For this review, take the finished solid that the model builds, in its own axes (mm). A direction names the side the tool comes from. Give positions to 0.01 mm unless a question says otherwise; leave off trailing zeros. Order: outer loops, then holes, each group sorted by start corner. A loop starts at its lowest first (then second) coordinate and runs counter-clockwise, first axis right, second up.
from build123d import *

# Parameters (mm, degrees)
F0_W     = 70
F0_H     = 50
F0_W_2   = 2.8157552083
F0_H_2   = 18.5818142361
F0_R     = 2.5
F1_DEPTH = 5


with BuildPart() as f1:
    # F0 (on Top) → F1 (new body)
    with BuildSketch(Plane.XY):
        with Locations((-35, 25)):
            Rectangle(F0_W, F0_H)
        Polygon((-58.9236111111, 34.7884114583), (-52.3589409722, 22.3914930556), (-45.7508680556, 34.7884114583), (-42.6312934028, 34.7884114583), (-50.9049479167, 19.6137152778), (-50.9049479167, 10), (-53.818359375, 10), (-53.818359375, 19.4780815972), (-62.0757378472, 34.7884114583), align=None, mode=Mode.SUBTRACT)
        with BuildLine():
            Line((-26.1328125, 10), (-28.2215711806, 10))
            Line((-28.2215711806, 10), (-28.7803819444, 12.6475694444))
            Line((-28.7803819444, 12.6475694444), (-28.916015625, 12.6475694444))
            add(Edge.make_bspline(
                [(-28.916015625, 12.6475694444), (-30.3049045139, 10.9006076389), (-31.6856553819, 10.2794053819)],
                knots=[0, 0, 0, 1, 1, 1], degree=2))
            add(Edge.make_bspline(
                [(-31.6856553819, 10.2794053819), (-33.06640625, 9.658203125), (-35.1388888889, 9.658203125)],
                knots=[0, 0, 0, 1, 1, 1], degree=2))
            add(Edge.make_bspline(
                [(-35.1388888889, 9.658203125), (-37.900390625, 9.658203125), (-39.4683159722, 11.0850694444)],
                knots=[0, 0, 0, 1, 1, 1], degree=2))
            add(Edge.make_bspline(
                [(-39.4683159722, 11.0850694444), (-41.0362413194, 12.5119357639), (-41.0362413194, 15.1378038194)],
                knots=[0, 0, 0, 1, 1, 1], degree=2))
            add(Edge.make_bspline(
                [(-41.0362413194, 15.1378038194), (-41.0362413194, 20.7638888889), (-32.0355902778, 21.03515625)],
                knots=[0, 0, 0, 1, 1, 1], degree=2))
            Line((-32.0355902778, 21.03515625), (-28.8834635417, 21.1382378472))
            Line((-28.8834635417, 21.1382378472), (-28.8834635417, 22.2938368056))
            add(Edge.make_bspline(
                [(-28.8834635417, 22.2938368056), (-28.8834635417, 24.4802517361), (-29.8220486111, 25.5219184028)],
                knots=[0, 0, 0, 1, 1, 1], degree=2))
            add(Edge.make_bspline(
                [(-29.8220486111, 25.5219184028), (-30.7606336806, 26.5635850694), (-32.8331163194, 26.5635850694)],
                knots=[0, 0, 0, 1, 1, 1], degree=2))
            add(Edge.make_bspline(
                [(-32.8331163194, 26.5635850694), (-35.1551649306, 26.5635850694), (-38.0848524306, 25.1421440972)],
                knots=[0, 0, 0, 1, 1, 1], degree=2))
            Line((-38.0848524306, 25.1421440972), (-38.9529079861, 27.2960069444))
            add(Edge.make_bspline(
                [(-38.9529079861, 27.2960069444), (-37.5802951389, 28.0392795139), (-35.9445529514, 28.4624565972)],
                knots=[0, 0, 0, 1, 1, 1], degree=2))
            add(Edge.make_bspline(
                [(-35.9445529514, 28.4624565972), (-34.3088107639, 28.8856336806), (-32.6595052083, 28.8856336806)],
                knots=[0, 0, 0, 1, 1, 1], degree=2))
            add(Edge.make_bspline(
                [(-32.6595052083, 28.8856336806), (-29.3391927083, 28.8856336806), (-27.7360026042, 27.4126519097)],
                knots=[0, 0, 0, 1, 1, 1], degree=2))
            add(Edge.make_bspline(
                [(-27.7360026042, 27.4126519097), (-26.1328125, 25.9396701389), (-26.1328125, 22.6844618056)],
                knots=[0, 0, 0, 1, 1, 1], degree=2))
            Line((-26.1328125, 22.6844618056), (-26.1328125, 10))
        make_face(mode=Mode.SUBTRACT)
        with Locations((-18.9306640625, 19.2909071181)):
            Rectangle(F0_W_2, F0_H_2, mode=Mode.SUBTRACT)
        with Locations((-41.0378689236, 42.0710678119)):
            Circle(F0_R, mode=Mode.SUBTRACT)
        with BuildLine():
            add(Edge.make_bspline(
                [(-20.1025390625, 32.2005208333), (-20.5772569444, 32.6671006944), (-20.5772569444, 33.6165364583)],
                knots=[0, 0, 0, 1, 1, 1], degree=2))
            add(Edge.make_bspline(
                [(-20.5772569444, 33.6165364583), (-20.5772569444, 34.5822482639), (-20.1025390625, 35.0325520833)],
                knots=[0, 0, 0, 1, 1, 1], degree=2))
            add(Edge.make_bspline(
                [(-20.1025390625, 35.0325520833), (-19.6278211806, 35.4828559028), (-18.9116753472, 35.4828559028)],
                knots=[0, 0, 0, 1, 1, 1], degree=2))
            add(Edge.make_bspline(
                [(-18.9116753472, 35.4828559028), (-18.2335069444, 35.4828559028), (-17.7425130208, 35.0244140625)],
                knots=[0, 0, 0, 1, 1, 1], degree=2))
            add(Edge.make_bspline(
                [(-17.7425130208, 35.0244140625), (-17.2515190972, 34.5659722222), (-17.2515190972, 33.6165364583)],
                knots=[0, 0, 0, 1, 1, 1], degree=2))
            add(Edge.make_bspline(
                [(-17.2515190972, 33.6165364583), (-17.2515190972, 32.6671006944), (-17.7425130208, 32.2005208333)],
                knots=[0, 0, 0, 1, 1, 1], degree=2))
            add(Edge.make_bspline(
                [(-17.7425130208, 32.2005208333), (-18.2335069444, 31.7339409722), (-18.9116753472, 31.7339409722)],
                knots=[0, 0, 0, 1, 1, 1], degree=2))
            add(Edge.make_bspline(
                [(-18.9116753472, 31.7339409722), (-19.6278211806, 31.7339409722), (-20.1025390625, 32.2005208333)],
                knots=[0, 0, 0, 1, 1, 1], degree=2))
        make_face(mode=Mode.SUBTRACT)
    extrude(amount=F1_DEPTH)


solid = f1.part
1) To check wall thickness, follow line 1 (X direction, y = 13, z = 0.6); line 2 (X direction, y = 29, z = 0.65); line 3 (X direction, y = 32.5, z = 1.3). State the ranges of each line that lie inside material, in increasing order.
Answer sheet:
line 1: x = -70 to -53.82, -50.9 to -40.71, -26.13 to -20.34, -17.52 to 0
line 2: x = -70 to -58.95, -55.86 to -48.84, -45.79 to 0
line 3: x = -70 to -60.84, -57.71 to -46.97, -43.88 to -20.33, -17.51 to 0
2) Clearance check with flat-ended pins moving along their axes: pin 1 (5 mm diameter, centred on x = -27, y = 34, fed in from -Z); pin 2 (3 mm diameter, centred on x = -41.04, y = 42.07, fed in from +Z). State where each tip first meets the part, or that it passes through.
Answer sheet:
pin 1: stops at z = 0
pin 2: passes through
3) We need section A-A on y = 43. Give the boundary of the cut face in (x, z), then the cut area to 3 significant figures.
Answer sheet:
outline: (-70, 0) - (-43.36, 0) - (-43.36, 5) - (-70, 5) - close; (-38.72, 0) - (0, 0) - (0, 5) - (-38.72, 5) - close
area: 327 mm2
4) Tool access review of faces 4 (the face through (-27, 10, 2)), 5 (the face through (-35, 25, 5)): name each direction out of +Z, -Z, +X, -X, +Y, -Y from which nothing blocks a thin tool from reaching the whole face with its end or side.
Answer sheet:
face 4: +Z, -Z
face 5: +Z, +X, -X, +Y, -Y
5) Draft analysis for pull direction X (two halves, no side actions). For faces 1 (the face through (-19, 10, 2)), 2 (the face through (-35, 25, 0)), 3 (the face through (-38.51, 26.2, 2.46)), state which applies: +X half, -X half, draft (parallel to the pull), parting line (faces both ways), or undercut.
Answer sheet:
face 1: undercut
face 2: draft
face 3: undercut
6) We need section B-B on x = -37. Count the separate pieces of the cut face and the enclosed holes in it, then the cut area to 3 significant figures.
Answer sheet:
separate pieces: 3
enclosed holes: 0
area: 185 mm2
